Source: CAD feature listing. Evaluate the final solid. Frame: model axes, mm. A direction names the side the tool comes from. Round coordinates to 2 decimals unless told otherwise and drop trailing zeros. Write each loop counter-clockwise with the first axis right and the second up, starting at its lowest first coordinate (ties: lowest second). Pieces come first, ordered by that corner, then holes. Notation, with made-up numbers: M 51,76.5 L 75,76.5 A27 cw 75,97.5 Z; hole C 62,35.5 d3. An arc over 180 degrees is marked long. Answer in a Markdown table with one row per item.
from build123d import *

# Parameters (mm, degrees)
SKETCH1_R           = 5
BOSS_EXTRUDE1_DEPTH = 10
CUT_EXTRUDE1_DEPTH  = 6.6
CHAMFER1_SIZE       = 0.5


with BuildPart() as part:
    # Sketch1 → Boss-Extrude1 (new body)
    with BuildSketch(Plane(origin=(0, 0, 0), x_dir=(1, 0, 0), z_dir=(0, 1, 0))):
        with Locations(Location((0, 0, 0), (0, 0, 270))):
            Circle(SKETCH1_R)
        Polygon((2.775, -1.602146997), (2.775, 1.602146997), (0, 3.204293994), (-2.775, 1.602146997), (-2.775, -1.602146997), (0, -3.204293994), align=None, mode=Mode.SUBTRACT)
        Polygon((0, -3.204293994), (2.775, -1.602146997), (2.775, 1.602146997), (0, 3.204293994), (-2.775, 1.602146997), (-2.775, -1.602146997), align=None)
    extrude(amount=BOSS_EXTRUDE1_DEPTH)

    # Sketch2 → Cut-Extrude1 (cut)
    with BuildSketch(Plane(origin=(0, 10, 0), x_dir=(1, 0, 0), z_dir=(0, 1, 0))):
        Polygon((-2.775, -1.602146997), (0, -3.204293994), (2.775, -1.602146997), (2.775, 1.602146997), (0, 3.204293994), (-2.775, 1.602146997), align=None)
    extrude(amount=-CUT_EXTRUDE1_DEPTH, mode=Mode.SUBTRACT)

    # Chamfer1
    chamfer1_edges = [part.edges().sort_by_distance(p)[0] for p in [
        (-2.775, 10, 0),
        (-1.3875, 10, 2.403220496),
        (1.3875, 10, 2.403220496),
        (2.775, 10, 0),
        (1.3875, 10, -2.403220496),
        (-1.3875, 10, -2.403220496),
    ]]
    chamfer(chamfer1_edges, length=CHAMFER1_SIZE)


solid = part.part
Q1. Material intervals for probe 1 along Y at (x, z) = (-2.25, -1.75); probe 2 along X at (y, z) = (7.75, -1.75); probe 3 along Z at (x, y) = (-2.5, 6.25), sorted ascending.
Solutions:
| item | result |
|---|---|
| probe 1 | y = 0 to 3.4 |
| probe 2 | x = -4.68 to -2.52, 2.52 to 4.68 |
| probe 3 | z = -4.33 to -1.76, 1.76 to 4.33 |
Q2. Access query for faces 4 (the flat face through (-1.534, 9.746, 2.603)), 5 (the flat face through (0, 0, 0)). Directions: +Z, -Z, +X, -X, +Y, -Y. A direction counts if a zero-diameter tool reaches every point of the face in a straight line with its end or side. Return the directions, or none.
Solutions:
| item | result |
|---|---|
| face 4 | +Y |
| face 5 | +Z, -Z, +X, -X, -Y |
Q3. Section A-A (y = 9). Return loops of the section in (x, z) (3 decimals), and give its area (3 significant figures).
Solutions:
| item | result |
|---|---|
| outline | C 0,0 d10; hole M -2.775,-1.602 L 0,-3.204 L 2.775,-1.602 L 2.775,1.602 L 0,3.204 L -2.775,1.602 Z |
| area | 51.9 mm2 |
Q4. Section D-D (y = 3). Return loops of the section in (x, z).
Solutions:
| item | result |
|---|---|
| outline | C 0,0 d10 |
Q5. Section C-C (x = 3). Return loops of the section in (y, z) (3 decimals), and give its area (3 significant figures).
Solutions:
| item | result |
|---|---|
| outline | M 0,-4 L 10,-4 L 10,-2.05 L 9.725,-1.732 L 9.725,1.732 L 10,2.05 L 10,4 L 0,4 Z |
| area | 79.0 mm2 |
Q6. Section B-B (z = 0). Return loops of the section in (x, y) (3 decimals), and give its area (3 significant figures).
Solutions:
| item | result |
|---|---|
| outline | M -5,0 L 5,0 L 5,10 L 3.275,10 L 2.775,9.5 L 2.775,3.4 L -2.775,3.4 L -2.775,9.5 L -3.275,10 L -5,10 Z |
| area | 63.1 mm2 |
Q7. Contact query for flat-ended pins moving along their axis: pin 1 Ø1 at (y, z) = (3, 3) entering from -X; pin 2 Ø3 at (x, z) = (0, 1) entering from +Y; pin 3 Ø1 at (y, z) = (2.5, -3.5) entering from -X. Output: stop coordinate, or through.
Solutions:
| item | result |
|---|---|
| pin 1 | stops at x = -4.33 |
| pin 2 | stops at y = 3.4 |
| pin 3 | stops at x = -4 |
Q8. Pull-direction query (Z, two-part tool) for faces 1 (the flat face through (1.2, 10, 3.3)), 2 (the cylindrical face through (-4.88, 4.93, -1.08)), 3 (the flat face through (1.368, 6.493, 2.414)); classes: pulls with the +Z half, pulls with the -Z half, needs draft (parallel to the pull), parting line crosses it, or undercut.
Solutions:
| item | result |
|---|---|
| face 1 | needs draft |
| face 2 | parting line crosses it |
| face 3 | undercut |
